For this review, use the dimensioned drawing (mm, ordinates from the lowest corner) and the shaded views. A direction names the side the tool comes from. Give positions to 0.01 mm unless a question says otherwise; leave off trailing zeros. Loops run counter-clockwise (first coordinate to the right, second up) from the corner with the lowest first, then second, coordinate; pieces in that order, holes last. Notation, with made-up numbers: (71.25, 66.25) - (90.25, 66.25) arc R12 ccw to (90.25, 75.25) - close; hole circle Ø1 at (12, 55.25). An arc over 180 degrees is marked (long way). Write each question's results on one line, items separated by ' | '.
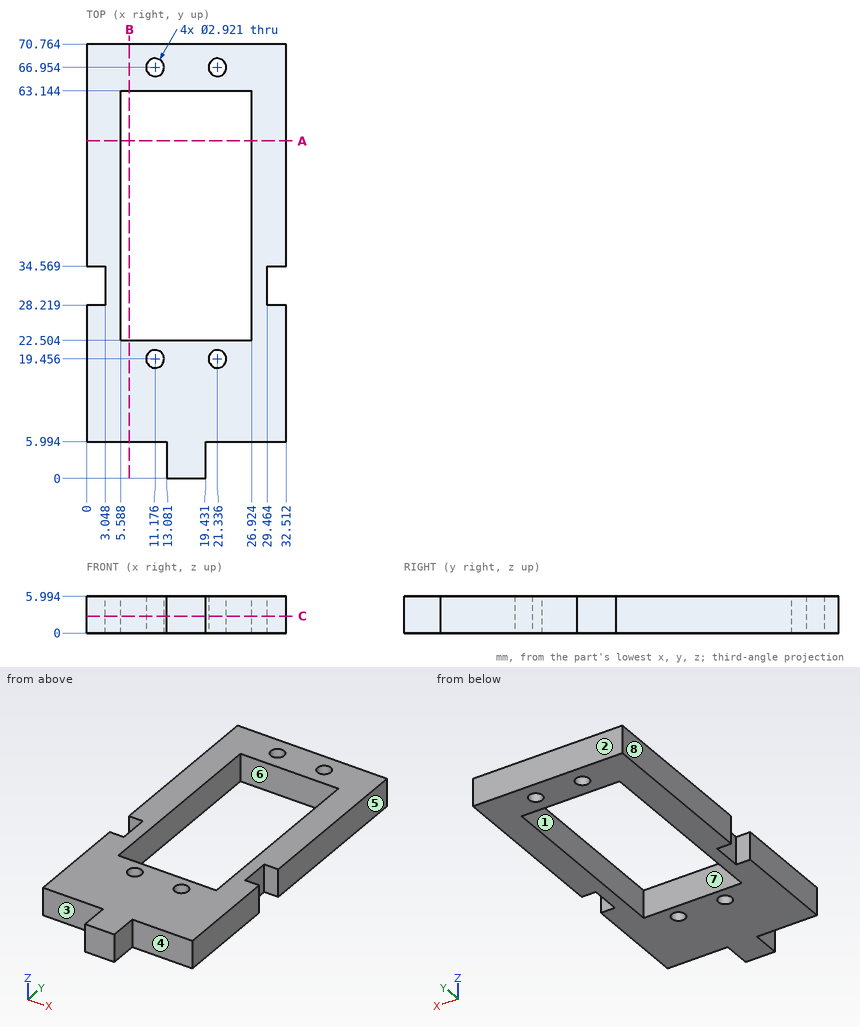
Item 1: We need section B-B on x = 7. Give the boundary of the cut face in (y, z) (1 decimal), then the cut area to 3 significant figures.
Output values:
outline: (6, 0) - (22.5, 0) - (22.5, 6) - (6, 6) - close; (63.1, 0) - (70.8, 0) - (70.8, 6) - (63.1, 6) - close | area: 145 mm²
Item 2: Clearance check with flat-ended pins moving along their axes: P1, Ø1.5, axis at x = 30.5, z = 2, coming from the -Y side; P2, Ø10, axis at x = 20.5, y = 35, coming from the -Z side; P3, Ø3, axis at y = 31, z = 3.5, coming from the -X side. State where each tip first meets the part, or that it passes through.
Output values:
P1: stops at y = 5.99 | P2: passes through | P3: stops at x = 3.05
Item 3: Tool access review of the marked faces 1, 2, 3 and 4: name each direction out of +Z, -Z, +X, -X, +Y, -Y from which nothing blocks a thin tool from reaching the whole face with its end or side.
Output values:
face 1: +Z, -Z | face 2: +Z, -Z, +X, -X, +Y | face 3: +Z, -Z, -X, -Y | face 4: +Z, -Z, +X, -Y
Item 4: Wall thickness on probe 1 along Y at (x, z) = (26, 5.05) (1 decimal); probe 2 along X at (y, z) = (49, 3.6); probe 3 along Y at (x, z) = (10, 0.7) (1 decimal): over which ranges is each line inside the solid? List them lowest first.
Output values:
probe 1: y = 6 to 22.5, 63.1 to 70.8 | probe 2: x = 0 to 5.59, 26.92 to 32.51 | probe 3: y = 6 to 18.6, 20.3 to 22.5, 63.1 to 66.1, 67.8 to 70.8
Item 5: We need section C-C on z = 2.8. Give the boundary of the cut face in (x, y) (1 decimal), then the cut area to 3 significant figures.
Output values:
outline: (0, 6) - (13.1, 6) - (13.1, 0) - (19.4, 0) - (19.4, 6) - (32.5, 6) - (32.5, 28.2) - (29.5, 28.2) - (29.5, 34.6) - (32.5, 34.6) - (32.5, 70.8) - (0, 70.8) - (0, 34.6) - (3, 34.6) - (3, 28.2) - (0, 28.2) - close; hole (5.6, 22.5) - (26.9, 22.5) - (26.9, 63.1) - (5.6, 63.1) - close; hole circle Ø2.9 at (11.2, 19.5); hole circle Ø2.9 at (11.2, 67); hole circle Ø2.9 at (21.3, 19.5); hole circle Ø2.9 at (21.3, 67) | area: 1,210 mm²
Item 6: We need section A-A on y = 55. Give the boundary of the cut face in (x, z) (1 decimal).
Output values:
outline: (0, 0) - (5.6, 0) - (5.6, 6) - (0, 6) - close; (26.9, 0) - (32.5, 0) - (32.5, 6) - (26.9, 6) - close
Item 7: Draft analysis for pull direction X (two halves, no side actions). For the marked faces 5, 6, 7 and 8, state which applies: +X half, -X half, draft (parallel to the pull), parting line (faces both ways), or undercut.
Output values:
face 5: +X half | face 6: undercut | face 7: undercut | face 8: -X half
